Can you work these out from the model? Positions are in its coordinate system, mm. Face numbers are marked on the shaded views. Coordinates: 2 decimals unless noted, no trailing zeros. Loops run counter-clockwise (first coordinate to the right, second up) from the corner with the lowest first, then second, coordinate; pieces in that order, holes last. Notation, with made-up numbers: (-11, 22.5) -> (42, 22.5) arc R11 ccw to (42, 33.5) -> close; hole circle Ø5 at (47, -40). An arc over 180 degrees is marked (long way). Put each result on its own line as item: value. Start each with the question number.
Item 1: We'd pull the mould along Y, two halves only. Please class the marked faces 1, 2, 3 and 4: pulls with the +Y half, pulls with the -Y half, needs draft (parallel to the pull), parting line crosses it, or undercut.
Item 2: Please list where these lines run through material, in increasing order: L1, parallel to Z at x = -3.5, y = 33; L2, parallel to X at y = -12.5, z = 20.25; L3, parallel to X at y = -23.5, z = 10.25. Write a range as from..to.
Item 3: If we section it at A-A on z = 16.75: Please give me the cut outline in (x, y).
Item 4: If we section it at B-B on z = 2: Please give me the cut outline in (x, y), plus the area to 3 significant figures.
Item 5: Will these pins go through, and if not, where does the flat tip stop? P1, Ø2, axis at x = 3, z = 4, coming from the -Y side; P2, Ø10, axis at x = -27, y = -13, coming from the +Z side; P3, Ø2, axis at y = -20.5, z = 13, coming from the -X side.
```python
from build123d import *

# Parameters (mm, degrees)
F1_DEPTH = 25.4
F2_R     = 53.6748278482
F3_DEPTH = 17.78
F4_R     = 17.77999


# Not quite as in the source:
# - a fillet or chamfer is up to 0.001 mm smaller than in the source, because OpenCascade refuses the exact size


with BuildPart() as f1:
    # F0 (on Top) → F1 (new body)
    with BuildSketch(Plane.XY):
        Polygon((58.9595362544, -28.3934161968), (58.9595362544, 28.3934161968), (14.5618028995, 63.799427074), (-40.8012650454, 51.1631680934), (-65.440148217, 0), (-40.8012650454, -51.1631680934), (14.5618028995, -63.799427074), align=None)
    extrude(amount=F1_DEPTH)

    # F2 (on face) → F3 (cut)
    with BuildSketch(Plane.XY.offset(25.4)):
        Circle(F2_R)
    extrude(amount=-F3_DEPTH, mode=Mode.SUBTRACT)

    # F4 (radius 17.78 in the source; OpenCascade refuses exactly that, so slightly less here)
    f4_edges = [f1.edges().sort_by_distance(p)[0] for p in [
        (-53.674828, 0, 7.62),
    ]]
    fillet(f4_edges, radius=F4_R)


solid = f1.part
```
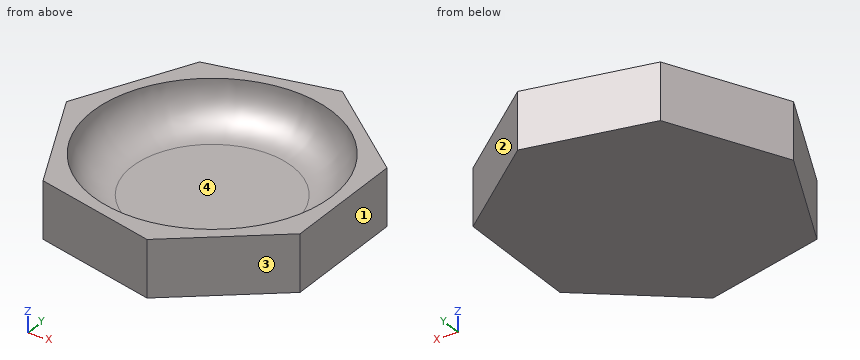
Solutions:
1. face 1: needs draft
1. face 2: pulls with the +Y half
1. face 3: pulls with the -Y half
1. face 4: undercut
2. L1: 0..7.62
2. L2: -59.42..-51.41, 51.41..58.96
2. L3: -54.12..-38.61, 38.61..58.96
3. outline: (-65.44, 0) -> (-40.8, -51.16) -> (14.56, -63.8) -> (58.96, -28.39) -> (58.96, 28.39) -> (14.56, 63.8) -> (-40.8, 51.16) -> close; hole circle Ø102.86 at (0, 0)
4. outline: (-65.44, 0) -> (-40.8, -51.16) -> (14.56, -63.8) -> (58.96, -28.39) -> (58.96, 28.39) -> (14.56, 63.8) -> (-40.8, 51.16) -> close
4. area: 11,700 mm^2
5. P1: y = -61.39
5. P2: z = 7.62
5. P3: x = -56.05
